from build123d import *

# Parameters (mm, degrees)
SKETCH2_W           = 84
SKETCH2_H           = 64
BOSS_EXTRUDE1_DEPTH = 3
SKETCH3_R           = 3.1
BOSS_EXTRUDE2_DEPTH = 2.5
SKETCH4_R           = 1.375
CUT_EXTRUDE1_DEPTH  = 95.667806042
SKETCH5_R           = 1.8
CUT_EXTRUDE2_DEPTH  = 95.555504868
FILLET1_R           = 9
FILLET2_R           = 9
CUT_EXTRUDE3_DEPTH  = 90.310693627
SKETCH7_W           = 2
SKETCH7_H           = 14
SKETCH7_W_2         = 3
SKETCH7_H_2         = 24
SKETCH7_W_3         = 4
SKETCH7_H_3         = 34
SKETCH7_W_4         = 24
SKETCH7_H_4         = 3
SKETCH7_W_5         = 34
SKETCH7_H_5         = 4
CUT_EXTRUDE4_DEPTH  = 90.310693627
FILLET3_R           = 1


# Some blends are built 0.0001 mm under size
with BuildPart() as part:
    # Sketch2 → Boss-Extrude1 (new body)
    with BuildSketch(Plane(origin=(0, 0, 0), x_dir=(1, 0, 0), z_dir=(0, 1, 0))):
        Rectangle(SKETCH2_W, SKETCH2_H)
        Polygon((-42, -32), (-42, -17), (-72.784271247, -47.784271247), (-60.284271247, -60.284271247), (-32, -32), align=None)
        Polygon((60.284271247, 60.284271247), (32, 32), (42, 32), (42, 17), (72.784271247, 47.784271247), align=None)
        Polygon((72.784271247, -47.784271247), (42, -17), (42, -32), (32, -32), (60.284271247, -60.284271247), align=None)
        Polygon((-42, 32), (-32, 32), (-60.284271247, 60.284271247), (-72.784271247, 47.784271247), (-42, 17), align=None)
    extrude(amount=BOSS_EXTRUDE1_DEPTH)

    # Sketch3 → Boss-Extrude2 (add)
    with BuildSketch(Plane(origin=(0, 3, 0), x_dir=(1, 0, 0), z_dir=(0, 1, 0))):
        with Locations(Location((-29, 24.5, 0), (0, 0, 270))):
            Circle(SKETCH3_R)
        with Locations(Location((-29, -24.5, 0), (0, 0, 270))):
            Circle(SKETCH3_R)
        with Locations(Location((29, -24.5, 0), (0, 0, 270))):
            Circle(SKETCH3_R)
        with Locations(Location((29, 24.5, 0), (0, 0, 270))):
            Circle(SKETCH3_R)
    extrude(amount=BOSS_EXTRUDE2_DEPTH)

    # Sketch4 → Cut-Extrude1 (cut, through all)
    with BuildSketch(Plane(origin=(0, 5.5, 0), x_dir=(1, 0, 0), z_dir=(0, 1, 0))):
        with Locations(Location((-29, 24.5, 0), (0, 0, 270))):
            Circle(SKETCH4_R)
        with Locations(Location((-29, -24.5, 0), (0, 0, 270))):
            Circle(SKETCH4_R)
        with Locations(Location((29, -24.5, 0), (0, 0, 270))):
            Circle(SKETCH4_R)
        with Locations(Location((29, 24.5, 0), (0, 0, 270))):
            Circle(SKETCH4_R)
    extrude(amount=-CUT_EXTRUDE1_DEPTH, mode=Mode.SUBTRACT)

    # Sketch5 → Cut-Extrude2 (cut, through all)
    with BuildSketch(Plane(origin=(0, 3, 0), x_dir=(1, 0, 0), z_dir=(0, 1, 0))):
        with Locations(Location((-57.5, 43.25, 0), (0, 0, 270))):
            Circle(SKETCH5_R)
        with Locations(Location((56, 43.25, 0), (0, 0, 270))):
            Circle(SKETCH5_R)
        with Locations(Location((56.75, -43.25, 0), (0, 0, 270))):
            Circle(SKETCH5_R)
        with Locations(Location((-56.75, -43.25, 0), (0, 0, 270))):
            Circle(SKETCH5_R)
    extrude(amount=-CUT_EXTRUDE2_DEPTH, mode=Mode.SUBTRACT)

    # Fillet1
    # the kernel refuses this fillet: 9 mm, written as the material it takes off along each edge
    with BuildSketch(Plane(origin=(-72.784271247, -22.5, 47.784271247), x_dir=(0.7071067811865487, 0, 0.7071067811865464), z_dir=(0, 1, 0)), Plane(origin=(-60.284271247, -22.5, 60.284271247), x_dir=(0.7071067811865467, 0, -0.7071067811865483), z_dir=(0, 1, 0)), Plane(origin=(60.284271247, -22.5, 60.284271247), x_dir=(0.7071067811865482, 0, -0.7071067811865467), z_dir=(0, 1, 0)), Plane(origin=(72.784271247, -22.5, 47.784271247), x_dir=(-0.7071067811865468, 0, -0.7071067811865483), z_dir=(0, 1, 0))) as fillet1_piece_1:
        with BuildLine():
            CenterArc((FILLET1_R, FILLET1_R), FILLET1_R, 180, 90)
            Line((0, FILLET1_R), (0, 0))
            Line((0, 0), (FILLET1_R, 0))
        make_face()
    extrude(amount=48, mode=Mode.SUBTRACT)
    with BuildSketch(Plane(origin=(72.784271247, -22.5, -47.784271247), x_dir=(-0.7071067811865472, 0, 0.707106781186548), z_dir=(0, 1, 0)), Plane(origin=(60.284271247, -22.5, -60.284271247), x_dir=(0.7071067811865487, 0, 0.7071067811865464), z_dir=(0, 1, 0)), Plane(origin=(-60.284271247, -22.5, -60.284271247), x_dir=(0.7071067811865467, 0, 0.7071067811865482), z_dir=(0, 1, 0)), Plane(origin=(-72.784271247, -22.5, -47.784271247), x_dir=(0.7071067811865491, 0, -0.7071067811865459), z_dir=(0, 1, 0))) as fillet1_piece_2:
        with BuildLine():
            CenterArc((FILLET1_R, -FILLET1_R), FILLET1_R, 90, 90)
            Line((0, -FILLET1_R), (0, 0))
            Line((0, 0), (FILLET1_R, 0))
        make_face()
    extrude(amount=48, mode=Mode.SUBTRACT)

    # Fillet2
    fillet2_edges = [part.edges().sort_by_distance(p)[0] for p in [
        (42, 1.5, 17),
        (32, 1.5, 32),
        (-32, 1.5, 32),
        (-42, 1.5, 17),
        (-42, 1.5, -17),
        (-32, 1.5, -32),
        (32, 1.5, -32),
        (42, 1.5, -17),
    ]]
    fillet(fillet2_edges, radius=FILLET2_R)

    # Sketch6 → Cut-Extrude3 (cut, through all)
    with BuildSketch(Plane(origin=(0, 3, 0), x_dir=(1, 0, 0), z_dir=(0, 1, 0))):
        Polygon((-24, 17), (-4, 17), (-18.699326173, -13), (-4, -13), (-4, -17), (-24, -17), (-9.300673827, 13), (-24, 13), align=None)
        Polygon((7, 13), (24, 13), (24, 17), (4, 17), (4, -17), (24, -17), (24, -13), (7, -13), align=None)
    extrude(amount=-CUT_EXTRUDE3_DEPTH, mode=Mode.SUBTRACT)

    # Sketch7 → Cut-Extrude4 (cut, through all)
    with BuildSketch(Plane(origin=(0, 3, 0), x_dir=(1, 0, 0), z_dir=(0, 1, 0))):
        with Locations((-39, 0)):
            Rectangle(SKETCH7_W, SKETCH7_H)
        with Locations((-34.5, 0)):
            Rectangle(SKETCH7_W_2, SKETCH7_H_2)
        with Locations((-28, 0)):
            Rectangle(SKETCH7_W_3, SKETCH7_H_3)
        with Locations((0, 28.5)):
            Rectangle(SKETCH7_W_4, SKETCH7_H_4)
        with Locations((0, 22)):
            Rectangle(SKETCH7_W_5, SKETCH7_H_5)
        with Locations((0, -22)):
            Rectangle(SKETCH7_W_5, SKETCH7_H_5)
        with Locations((0, -28.5)):
            Rectangle(SKETCH7_W_4, SKETCH7_H_4)
        with Locations((28, 0)):
            Rectangle(SKETCH7_W_3, SKETCH7_H_3)
        with Locations((34.5, 0)):
            Rectangle(SKETCH7_W_2, SKETCH7_H_2)
        with Locations((39, 0)):
            Rectangle(SKETCH7_W, SKETCH7_H)
    extrude(amount=-CUT_EXTRUDE4_DEPTH, mode=Mode.SUBTRACT)

    # Fillet3
    fillet3_edges = [part.edges().sort_by_distance(p)[0] for p in [
        (-12, 1.5, -27),
        (12, 1.5, -27),
        (17, 1.5, -20),
        (-17, 1.5, -20),
        (-17, 1.5, -24),
        (17, 1.5, -24),
        (12, 1.5, -30),
        (-12, 1.5, -30),
        (-17, 1.5, 20),
        (17, 1.5, 20),
        (17, 1.5, 24),
        (12, 1.5, 30),
        (-12, 1.5, 30),
        (-17, 1.5, 24),
        (30, 1.5, 17),
        (36, 1.5, 12),
        (40, 1.5, 7),
        (38, 1.5, 7),
        (33, 1.5, 12),
        (26, 1.5, 17),
        (26, 1.5, -17),
        (33, 1.5, -12),
        (38, 1.5, -7),
        (30, 1.5, -17),
        (36, 1.5, -12),
        (40, 1.5, -7),
        (-30, 1.5, 17),
        (-26, 1.5, 17),
        (-30, 1.5, -17),
        (-26, 1.5, -17),
        (-33, 1.5, -12),
        (-36, 1.5, -12),
        (-33, 1.5, 12),
        (-36, 1.5, 12),
        (-38, 1.5, 7),
        (-40, 1.5, 7),
        (-38, 1.5, -7),
        (-40, 1.5, -7),
    ]]
    fillet(fillet3_edges, radius=FILLET3_R - 0.0001)  # a hair under: the kernel refuses the full size


solid = part.part
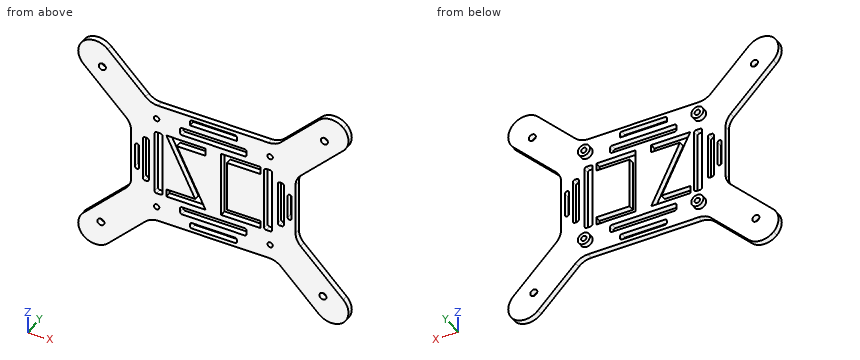
The listing builds one solid part. Answer for the finished solid, in the listing's coordinates (mm). Coordinates: 2 decimals unless noted, no trailing zeros. Write each loop counter-clockwise with the first axis right and the second up, starting at its lowest first coordinate (ties: lowest second). Pieces come first, ordered by that corner, then holes. Notation, with made-up numbers: (-1.5, -34) - (49.5, -34) arc R18 cw to (49.5, -25) - close; hole circle Ø1 at (13.5, 26.25). An arc over 180 degrees is marked (long way). Put each result on its own line as item: value.
1. The part is cut by section D-D on x = -21. Give the vertices of the cut face in (y, z), plus the area to 3 significant figures.
Answer sheet:
outline: (0, -32) - (3, -32) - (3, -17) - (0, -17) - close; (0, -13) - (3, -13) - (3, 10.88) - (0, 10.88) - close; (0, 17) - (3, 17) - (3, 32) - (0, 32) - close
area: 162 mm^2
2. Flat-ended cylindrical pins translate along their axes: pin 1 Ø0.9 at (y, z) = (1, 5) entering from -X; pin 2 Ø4 at (x, z) = (-57.5, -43.25) entering from -Y; pin 3 Ø2 at (x, y) = (33.5, 1) entering from +Z; pin 4 Ø1 at (x, z) = (41.5, 18.5) entering from +Y. Find the tip coordinate at first contact, or state that the pin passes through.
Answer sheet:
pin 1: stops at x = -42
pin 2: stops at y = 0
pin 3: stops at z = 34.5
pin 4: stops at y = 3
3. The part is cut by section B-B on z = -43.25. Give the vertices of the cut face in (x, y), plus the area to 3 significant figures.
Answer sheet:
outline: (-67.83, 0) - (-59.3, 0) - (-59.3, 3) - (-67.83, 3) - close; (-55.7, 0) - (-43.25, 0) - (-43.25, 3) - (-55.7, 3) - close; (43.25, 0) - (54.2, 0) - (54.2, 3) - (43.25, 3) - close; (57.8, 0) - (67.83, 0) - (67.83, 3) - (57.8, 3) - close
area: 126 mm^2
4. The part is cut by section A-A on x = 1. Give the vertices of the cut face in (y, z), plus the area to 3 significant figures.
Answer sheet:
outline: (0, -32) - (3, -32) - (3, -30) - (0, -30) - close; (0, -27) - (3, -27) - (3, -24) - (0, -24) - close; (0, -20) - (3, -20) - (3, 20) - (0, 20) - close; (0, 24) - (3, 24) - (3, 27) - (0, 27) - close; (0, 30) - (3, 30) - (3, 32) - (0, 32) - close
area: 150 mm^2
5. The part is cut by section C-C on y = 1.4. State how many separate pieces and enclosed holes the cut face has, plus the area to 3 significant figures.
Answer sheet:
separate pieces: 1
enclosed holes: 20
area: 6,480 mm^2
6. Find the intervals of material crossed by line 1 along Z through (x, y) = (1, 2.55); line 2 along Z through (x, y) = (4.5, 0.5); line 3 along X through (y, z) = (3.95, 24.5) (3 decimals), in increasing order. Write a range as from..to.
Answer sheet:
line 1: z = -32..-30, -27..-24, -20..20, 24..27, 30..32
line 2: z = -32..-30, -27..-24, -20..-17, 17..20, 24..27, 30..32
line 3: x = -32.1..-30.375, -27.625..-25.9, 25.9..27.625, 30.375..32.1
